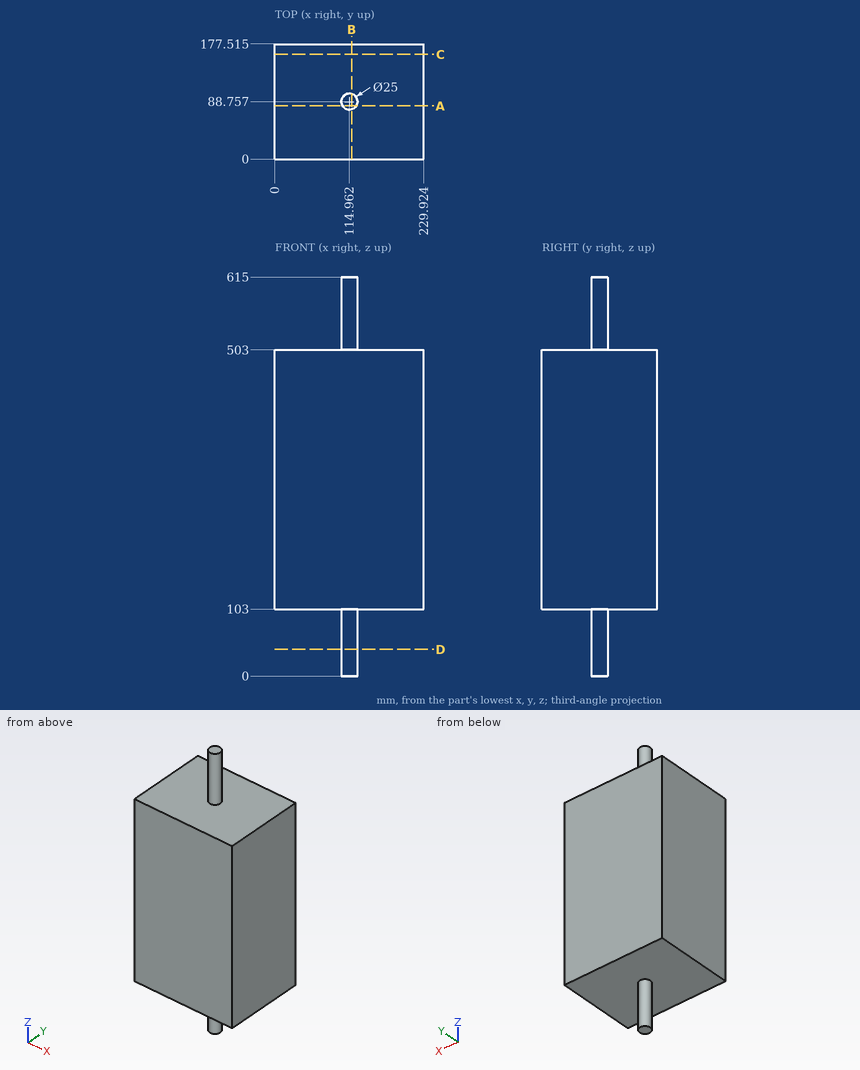
The figure shows three views and two pictorial views of one solid part (mm, origin at its lowest corner). Answer the questions. Give positions to 0.01 mm unless a question says otherwise; leave off trailing zeros. Order: outer loops, then holes, each group sorted by start corner. A loop starts at its lowest first (then second) coordinate and runs counter-clockwise, first axis right, second up. Notation, with made-up numbers: M -24,47 L -4,47 A18 ccw -4,70 Z; hole C 81,77.25 d4. An arc over 180 degrees is marked long. Return JSON: item names as keys, results as strings.
Q1. Find section C-C, the plane y = 161.5. Write down the section's boundary in (x, z), and give its area (3 significant figures).
Answer below:
{"outline": "M 0,103 L 229.92,103 L 229.92,503 L 0,503 Z", "area": "92,000 mm^2"}
Q2. Find section B-B, the plane x = 118.5. Write down the section's boundary in (y, z) (1 decimal), and give its area (3 significant figures).
Answer below:
{"outline": "M 0,103 L 76.8,103 L 76.8,0 L 100.7,0 L 100.7,103 L 177.5,103 L 177.5,503 L 100.7,503 L 100.7,615 L 76.8,615 L 76.8,503 L 0,503 Z", "area": "76,200 mm^2"}
Q3. Find section A-A, the plane y = 82. Write down the section's boundary in (x, z).
Answer below:
{"outline": "M 0,103 L 104.45,103 L 104.45,0 L 125.48,0 L 125.48,103 L 229.92,103 L 229.92,503 L 125.48,503 L 125.48,615 L 104.45,615 L 104.45,503 L 0,503 Z"}
Q4. Each of these flat-tipped pins is pushed along its axis until it touches: pin 1 (1.5 mm diameter, centred on x = 181.5, z = 121.5, fed in from -Y); pin 2 (6 mm diameter, centred on x = 191, y = 110.5, fed in from +Z); pin 3 (12 mm diameter, centred on x = 53, y = 126.5, fed in from -Z). Where does it stop, or does it pass through?
Answer below:
{"pin 1": "stops at y = 0", "pin 2": "stops at z = 503", "pin 3": "stops at z = 103"}
Q5. Find section D-D, the plane z = 41. Write down the section's boundary in (x, y), and give its area (3 significant figures).
Answer below:
{"outline": "C 114.96,88.76 d25", "area": "491 mm^2"}
Q6. Find the intervals of material crossed by line 1 along Z through (x, y) = (104, 156), in increasing order. Write a range as [from, to].
Answer below:
{"line 1": "z = [103, 503]"}
